Work out the finished part from the listing and answer in its coordinate system (mm). Face numbers are marked on the shaded views. A direction names the side the tool comes from. Coordinates: 2 decimals unless noted, no trailing zeros. Write each loop counter-clockwise with the first axis right and the second up, starting at its lowest first coordinate (ties: lowest second). Pieces come first, ordered by that corner, then holes. Notation, with made-up numbers: M 12,2 L 47,2 A15 ccw 47,13 Z; hole C -6,3 d2. An arc over 180 degrees is marked long. Answer as CSV lines item,"result". Start each with the question number.
(1) The mould has two halves that part along X. Classify the marked faces 1, 2, 3 and 4: released by +X, released by -X, zero draft, split by the parting line, or undercut.
(2) Flat-ended cylindrical pins translate along their axes: P1, Ø1.1, axis at y = 4.5, z = -0.5, coming from the +X side; P2, Ø1.1, axis at y = 4.5, z = 1.5, coming from the -X side; P3, Ø6, axis at y = 6.5, z = -1, coming from the +X side. Find the tip coordinate at first contact, or state that the pin passes through.
(3) For the marked faces 5, 6, 7 and 8, determine the directions among +Z, -Z, +X, -X, +Y, -Y from which every point of the face is accessible in a straight line to the end or side of a thin tool.
(4) A cutting plane is placed at A-A on x = 4. Give the vertices of the cut face in (y, z), then the cut area to 3 significant figures.
(5) A cutting plane is placed at B-B on z = -0.5. Give the vertices of the cut face in (x, y).
(6) A cutting plane is placed at D-D on z = 4.25. Give the vertices of the cut face in (x, y).
(7) Find the intervals of material crossed by L1, parallel to Z at x = 4, y = 1.1; L2, parallel to Y at x = 32.5, z = 1.5; L3, parallel to X at y = 2.15, z = 0, in increasing order. Write a range as [from, to].
(8) A cutting plane is placed at C-C on y = 2.25. Give the vertices of the cut face in (x, z).
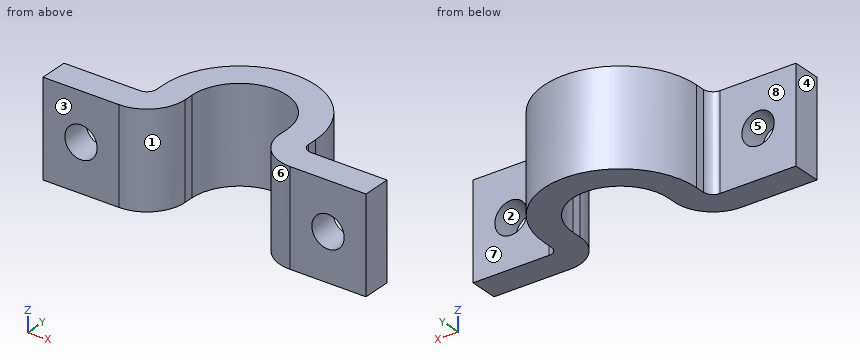
Autodesk Inventor part; units mm, degrees
ref_plane "YZ Plane" through (0, 0, 0) normal (1, 0, 0) x (0, 1, 0)
ref_plane "XZ Plane" through (0, 0, 0) normal (0, 1, 0) x (-1, 0, 0)
ref_plane "XY Plane" through (0, 0, 0) normal (0, 0, 1) x (1, 0, 0)
sketch "Sketch1" plane through (0, 0, 0) normal (0, 0, 1) x (1, 0, 0)
  line L0 (0, 0) -> (12, 0)
  line L1 (12, 0) -> (12, 3)
  line L2 (12, 3) -> (0, 3)
  line L3 (0, 3) -> (0, 0)
  line L4 (12, 0) -> (9, 0)
  line L5 (9, 0) -> (9, 5)
  line L6 (9, 5) -> (12, 5)
  line L7 (12, 5) -> (12, 0)
  line L8 (22, 5) -> (25, 5)
  line L9 (25, 5) -> (25, 0)
  line L10 (25, 0) -> (22, 0)
  line L11 (22, 0) -> (22, 5)
  line L12 (22, 0) -> (34, 0)
  line L13 (34, 0) -> (34, 3)
  line L14 (34, 3) -> (22, 3)
  line L15 (22, 3) -> (22, 0)
  arc A0 (25, 5) -> (9, 5) centre (17, 5) ccw
  arc A1 (22, 5) -> (12, 5) centre (17, 5) ccw
  dimension "d0" = 3
  dimension "d1" = 3
  dimension "d2" = 12
  dimension "d3" = 12
  dimension "d4" = 5
  dimension "d5" = 5
extrude "Extrusion1" add sketch "Sketch1" along normal mid plane 10
fillet "Fillet1" radius 1 2 edges at (25, 3, 0) (9, 3, 0)
fillet "Fillet2" radius 4 2 edges at (22, 0, 0) (12, 0, 0)
sketch "Sketch2" plane through (0, 3, 5) normal (0, 1, 0) x (1, 0, 0)
  line L0 (0, 10) -> (0, 0)
  line L1 (0, 10) -> (8, 10)
  line L2 (26, 10) -> (34, 10)
  point P0 (0, 5)
  point P1 (4, 5)
  point P2 (30, 5)
  point P3 (0, 5)
  point P4 (4, 10)
  point P5 (30, 10)
  dimension "d10" = 26
hole "Hole1" at (4, 3, 0) at (30, 3, 0) direction (0, -1, 0) diameter 3.4 end through all
equation "\"d1\" = d0"
equation "\"d3\" = d2"
properties part number "Top_Cable Tie" material "Aluminum 6061"
Here are the results:
1,face 1,"undercut"
1,face 2,"undercut"
1,face 3,"zero draft"
1,face 4,"released by -X"
2,P1,"stops at x = 25"
2,P2,"stops at x = 9"
2,P3,"stops at x = 25.13"
3,face 5,"+Y, -Y"
3,face 6,"+Z, -Z, -Y"
3,face 7,"+Z, -Z, +X, +Y"
3,face 8,"+Z, -Z, -X, +Y"
4,outline,"M 0,-5 L 3,-5 L 3,-1.7 L 0,-1.7 Z; M 0,1.7 L 3,1.7 L 3,5 L 0,5 Z"
4,area,"19.8 mm^2"
5,outline,"M 0,0 L 2.38,0 L 2.38,3 L 0,3 Z; M 5.62,0 L 8,0 A4 ccw 12,4 L 12,5 A5 cw 22,5 L 22,4 A4 ccw 26,0 L 28.38,0 L 28.38,3 L 26,3 A1 cw 25,4 L 25,5 A8 ccw 9,5 L 9,4 A1 cw 8,3 L 5.62,3 Z; M 31.62,0 L 34,0 L 34,3 L 31.62,3 Z"
6,outline,"M 0,0 L 8,0 A4 ccw 12,4 L 12,5 A5 cw 22,5 L 22,4 A4 ccw 26,0 L 34,0 L 34,3 L 26,3 A1 cw 25,4 L 25,5 A8 ccw 9,5 L 9,4 A1 cw 8,3 L 0,3 Z"
7,L1,"z = [-5, -1.7], [1.7, 5]"
7,L2,"y = [0, 3]"
7,L3,"x = [0, 2.3], [5.7, 11.55], [22.45, 28.3], [31.7, 34]"
8,outline,"M 0,-5 L 11.6,-5 L 11.6,5 L 0,5 Z; M 22.4,-5 L 34,-5 L 34,5 L 22.4,5 Z; hole C 4,0 d3.4; hole C 30,0 d3.4"
